Part model, mm, in its own coordinate system. Face numbers are marked on the shaded views. Give positions to 0.01 mm unless a question says otherwise; leave off trailing zeros. Order: outer loops, then holes, each group sorted by start corner. A loop starts at its lowest first (then second) coordinate and runs counter-clockwise, first axis right, second up.
1. Slice it at C-C on x = 60. List the corners of the cut face in (y, z), and give its area (3 significant figures).
2. Probe line 1 (Y direction, x = 63, z = 2.05); line 2 (X direction, y = 4, z = -1.9); line 3 (X direction, y = 1.5, z = -1.9). List the from-to ranges inside material, lowest first.
3. Slice it at B-B on z = 1.5. List the corners of the cut face in (x, y), and give its area (3 significant figures).
4. Mould opens along X. For the marked faces 1, 2, 3 and 4 say: +X half, -X half, draft (parallel to the pull), parting line (faces both ways), or undercut.
5. Slice it at A-A on x = 63. List the corners of the cut face in (y, z), and give its area (3 significant figures).
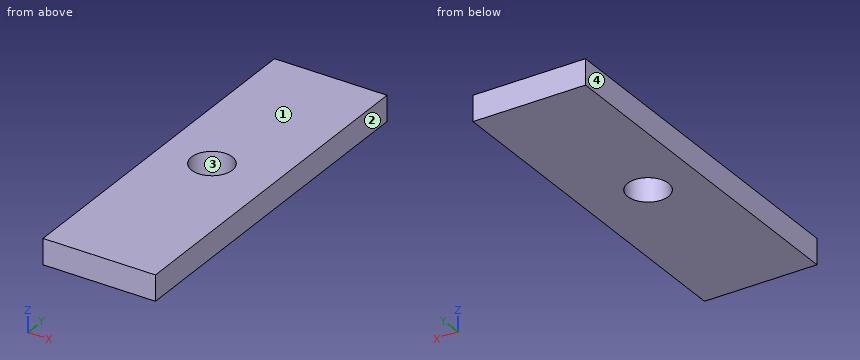
from build123d import *

# Parameters (mm, degrees)
SKETCH1_W           = 150
SKETCH1_H           = 70
BOSS_EXTRUDE1_DEPTH = 2.5
SKETCH2_R           = 4
CUT_EXTRUDE1_DEPTH  = 6
SKETCH3_W           = 120
SKETCH3_H           = 70
CUT_EXTRUDE2_DEPTH  = 6
SKETCH4_W           = 8
SKETCH4_H           = 70
CUT_EXTRUDE3_DEPTH  = 6


with BuildPart() as part:
    # Sketch1 → Boss-Extrude1 (new body, symmetric)
    with BuildSketch(Plane.XY):
        Rectangle(SKETCH1_W, SKETCH1_H)
    extrude(amount=BOSS_EXTRUDE1_DEPTH, both=True)

    # Sketch2 → Cut-Extrude1 (cut, through all)
    with BuildSketch(Plane.XY.offset(2.5)):
        with Locations((63, 0.628549325)):
            Circle(SKETCH2_R)
        with Locations((29.001496193, 0.309583996)):
            Circle(SKETCH2_R)
        with Locations((-42.995335398, -0.365871995)):
            Circle(SKETCH2_R)
        with Locations((-3.99705162, 0)):
            Circle(SKETCH2_R)
    extrude(amount=-CUT_EXTRUDE1_DEPTH, mode=Mode.SUBTRACT)

    # Sketch3 → Cut-Extrude2 (cut, through all)
    with BuildSketch(Plane(origin=(0, 0, -2.5), x_dir=(-1, 0, 0), z_dir=(0, 0, -1))):
        with Locations((15, 0)):
            Rectangle(SKETCH3_W, SKETCH3_H)
    extrude(amount=-CUT_EXTRUDE2_DEPTH, mode=Mode.SUBTRACT)

    # Sketch4 → Cut-Extrude3 (cut, through all)
    with BuildSketch(Plane(origin=(0, 0, -2.5), x_dir=(-1, 0, 0), z_dir=(0, 0, -1))):
        with Locations((-49, 0)):
            Rectangle(SKETCH4_W, SKETCH4_H)
    extrude(amount=-CUT_EXTRUDE3_DEPTH, mode=Mode.SUBTRACT)


solid = part.part
Data:
1. outline: (-35, -2.5) - (-2.02, -2.5) - (-2.02, 2.5) - (-35, 2.5) - close; (3.27, -2.5) - (35, -2.5) - (35, 2.5) - (3.27, 2.5) - close
1. area: 324 mm2
2. line 1: y = -35 to -3.37, 4.63 to 35
2. line 2: x = 53 to 60.85, 65.15 to 75
2. line 3: x = 53 to 59.1, 66.9 to 75
3. outline: (53, -35) - (75, -35) - (75, 35) - (53, 35) - close; hole circle Ø8 at (63, 0.63)
3. area: 1,490 mm2
4. face 1: draft
4. face 2: +X half
4. face 3: undercut
4. face 4: -X half
5. outline: (-35, -2.5) - (-3.37, -2.5) - (-3.37, 2.5) - (-35, 2.5) - close; (4.63, -2.5) - (35, -2.5) - (35, 2.5) - (4.63, 2.5) - close
5. area: 310 mm2
